Could you check a few things on this model? Use its own coordinates, in mm. A direction names the side the tool comes from. Coordinates: 2 decimals unless noted, no trailing zeros. Order: outer loops, then holes, each group sorted by start corner. A loop starts at its lowest first (then second) coordinate and runs counter-clockwise, first axis right, second up. Notation, with made-up numbers: M 70.5,6.5 L 97.5,6.5 A11 cw 97.5,16.5 Z; hole C -34.5,-24 d2. An arc over 180 degrees is marked long. Write item = value, one per line. Start each with the question number.
Autodesk Inventor part; units mm, degrees
ref_plane "YZ Plane" through (0, 0, 0) normal (1, 0, 0) x (0, 1, 0)
ref_plane "XZ Plane" through (0, 0, 0) normal (0, 1, 0) x (-1, 0, 0)
ref_plane "XY Plane" through (0, 0, 0) normal (0, 0, 1) x (1, 0, 0)
sketch "Sketch3" plane through (0, 0, 0) normal (0, 1, 0) x (-1, 0, 0)
  arc A0 (0, 0) -> (-0.5498, 50.794) centre (-0.5498, 25.394) ccw
  arc A1 (37.5561, -8.2003) -> (-0.5498, 76.194) centre (-0.5498, 25.394) ccw
  line L0 (0, 0) -> (-53.975, 0)
  line L1 (-53.975, 0) -> (-53.975, -50.8)
  line L2 (-53.975, -50.8) -> (0, -50.8)
  line L3 (0, -50.8) -> (37.5561, -8.2003)
  line L4 (-0.5498, 76.194) -> (-0.5498, 50.794)
  line L5 (50.2502, 25.394) -> (37.5502, 25.394)
  circle A2 centre (37.5502, 25.394) radius 2.3812
  line L6 (24.8487, 25.6689) -> (12.1517, 25.394)
  line L7 (12.1517, 25.394) -> (12.1517, 85.7885)
  line L8 (12.1517, 85.7885) -> (12.1517, 25.394)
  line L9 (12.1517, 25.394) -> (12.1517, -39.1077)
  line L10 (-0.5498, 63.494) -> (12.1517, 63.494)
  line L11 (12.1517, 3.3979) -> (12.1517, -37.0164)
  line L12 (12.1517, -16.8093) -> (14.0122, -16.8093)
  circle A3 centre (12.1517, -16.8093) radius 2.3812
  circle A4 centre (12.1517, 63.494) radius 2.3812
  dimension "d19" = 25.4
  dimension "d20" = 25.4
  dimension "d21" = 53.975
  dimension "d22" = 50.8
  dimension "d23" = 53.975
  dimension "d39" = 12.7
  dimension "d40" = 4.7625
  dimension "d42" = 12.7
  dimension "d43" = 4.7625
  dimension "d44" = 4.7625
extrude "Extrusion3" add sketch "Sketch3" along normal blind 3.175 contours A0 L9 A3 L3 L2 L1 L0 | A2 | A0 L7 A4 A1 L3 L9 A3 | A3 L9 | L9 A3 | A0 L4 L10 A4 L7 | A4 L10 L7 | L7 A4 | L4 A1 L7 A4 L10 | L10 A4 L7
fillet "Fillet3" radius 3.175 5 edges at (0, 1.5875, -50.8) (53.975, 1.5875, -50.8) (53.975, 1.5875, 0) (0.5498, 1.5875, 50.794) (0.5498, 1.5875, 76.194)
sketch "Sketch4" plane through (0, 3.175, 0) normal (0, 1, 0) x (1, 0, 0)
  line L0 (53.975, 3.175) -> (53.975, 47.625)
  line L1 (53.975, 25.4) -> (41.275, 25.4)
  line L2 (41.275, 25.4) -> (41.275, 38.1)
  line L3 (41.275, 38.1) -> (41.275, 12.7)
  line L4 (41.275, 12.7) -> (15.875, 12.7)
  point P0 (0, 0)
  point P1 (15.875, 38.1)
  dimension "d27" = 12.7
  dimension "d28" = 12.7
  dimension "d29" = 25.4
  dimension "d30" = 25.4
  dimension "d31" = 25.4
hole "Hole1" at (15.875, 3.175, -38.1) at (15.875, 3.175, -12.7) at (41.275, 3.175, -12.7) at (41.275, 3.175, -38.1) direction (0, -1, 0) diameter 4.7625 end through all
extrude "Extrusion4" cut sketch "Sketch3" along normal blind 3.175 contours A2 | A3 L9 | L9 A3 | A4 L10 L7 | L7 A4 | L10 A4 L7
properties part number "hook v2"
(1) Thinking about a two-plate mould opening in Z: for faces 1 (the cylindrical face through (-13.25, 1.565, -14.697)), 2 (the flat face through (-19, 1.57, -29.25)), 3 (the cylindrical face through (-46.1, 1.6, 45.5)), which applies, released by +Z, released by -Z, zero draft, split by the parting line, or undercut?
(2) Imagine slicing it at D-D on z = -38.1. List the corners of the cut face in (x, y) for me (3 decimals).
(3) For faces 4 (the flat face through (0.55, 2, 63)), 5 (the cylindrical face through (-0.237, 1.61, 51.7)), 6 (the cylindrical face through (-38.649, 1.565, 27.507)), which set-ups out of +Z, -Z, +X, -X, +Y, -Y let a thin tool reach every point of the face, with its end or its side?
(4) Imagine slicing it at A-A on z = -12.7. List the corners of the cut face in (x, y) for me (3 decimals).
(5) Imagine slicing it at C-C on x = -12. List the corners of the cut face in (y, z) for me (3 decimals).
(6) Please list where these lines run through material, in increasing order: probe 1 along Z at (x, y) = (41.5, 2.7); probe 2 along X at (y, z) = (2.1, -13.5) (3 decimals); probe 3 along Z at (x, y) = (34, 0.4). Write a range as from..to.
(7) Will these pins go through, and if not, where does the flat tip stop? P1, Ø3, axis at x = 41.275, z = -38.1, coming from the +Y side; P2, Ø1, axis at x = 14.5, y = 2, coming from the +Z side; P3, Ø1, axis at x = -18.5, y = 1.5, coming from the +Z side.
(8) Imagine slicing it at B-B on y = 1.7. Give the number of separate pieces and of enclosed holes in the cut face, plus the area to 3 significant figures.
Response:
q1.face_1 = undercut
q1.face_2 = released by -Z
q1.face_3 = split by the parting line
q2.outline = M -11.196,0 L 13.494,0 L 13.494,3.175 L -11.196,3.175 Z; M 18.256,0 L 38.894,0 L 38.894,3.175 L 18.256,3.175 Z; M 43.656,0 L 53.975,0 L 53.975,3.175 L 43.656,3.175 Z
q3.face_4 = +Z, +X, +Y, -Y
q3.face_5 = +X, +Y, -Y
q3.face_6 = +Y, -Y
q4.outline = M -33.589,0 L 13.494,0 L 13.494,3.175 L -33.589,3.175 Z; M 18.256,0 L 38.894,0 L 38.894,3.175 L 18.256,3.175 Z; M 43.656,0 L 53.975,0 L 53.975,3.175 L 43.656,3.175 Z
q5.outline = M 0,-37.188 L 3.175,-37.188 L 3.175,-19.186 L 0,-19.186 Z; M 0,-14.433 L 3.175,-14.433 L 3.175,3.311 L 0,3.311 Z; M 0,47.477 L 3.175,47.477 L 3.175,61.118 L 0,61.118 Z; M 0,65.87 L 3.175,65.87 L 3.175,74.619 L 0,74.619 Z
q6.probe_1 = -50.8..-40.47, -35.73..-15.07, -10.33..0
q6.probe_2 = -32.884..13.632, 18.118..39.032, 43.518..53.975
q6.probe_3 = -50.8..0
q7.P1 = through
q7.P2 = 0
q7.P3 = 72.69
q8.separate_pieces = 1
q8.enclosed_holes = 7
q8.area = 5,990 mm2
